Autodesk Inventor part; units mm, degrees
ref_plane "YZ Plane" through (0, 0, 0) normal (1, 0, 0) x (0, 1, 0)
ref_plane "XZ Plane" through (0, 0, 0) normal (0, 1, 0) x (-1, 0, 0)
ref_plane "XY Plane" through (0, 0, 0) normal (0, 0, 1) x (1, 0, 0)
sketch "Sketch1" plane through (0, 0, 0) normal (0, 0, 1) x (1, 0, 0)
  circle A0 centre (0, 0) radius 3.175
  circle A1 centre (0, 0) radius 1.5875
  dimension "d0" = 6.35
  dimension "d1" = 3.175
extrude "Extrusion1" add sketch "Sketch1" along normal blind 2.3813
sketch "Sketch2" plane through (0, 0, 2.3813) normal (0, 0, 1) x (1, 0, 0)
  circle A0 centre (0, 0) radius 1.905
  circle A1 centre (0, 0) radius 2.8575
  dimension "d4" = 3.81
  dimension "d5" = 5.715
extrude "Extrusion2" cut sketch "Sketch2" against normal blind 0.127
sketch "Sketch3" plane through (0, 0, 0) normal (0, 0, -1) x (-1, 0, 0)
  circle A0 centre (0, 0) radius 2.8575
  circle A1 centre (0, 0) radius 1.905
extrude "Extrusion3" cut sketch "Sketch3" against normal blind 0.127
properties part number "bearing_1_8inch" material "Stainless Steel"
Could you check a few things on this model? Use its own coordinates, in mm. A direction names the side the tool comes from. Give positions to 0.01 mm unless a question says otherwise; leave off trailing zeros. Write each loop counter-clockwise with the first axis right and the second up, starting at its lowest first coordinate (ties: lowest second). Pieces come first, ordered by that corner, then holes. Notation, with made-up numbers: (-31.5, 83.5) -> (15.5, 83.5) arc R17 ccw to (15.5, 87.5) -> close; hole circle Ø11 at (72, 55). An arc over 180 degrees is marked (long way). Answer as CSV lines item,"result". Start each with the question number.
(1) I'm going to push flat-ended pins straight in: pin 1 Ø1.7 at (x, y) = (1, -0.5) entering from -Z; pin 2 Ø1 at (y, z) = (-2, 0.5) entering from -X. Where does each tip first touch, or does it pass through?
(2) If we mould it in two halves opening along X, with no side actions, what happens to faces 1 (the face through (-0.69, 3.1, 1.17)), 2 (the face through (-1, -2, 0.127))? For each: +X half, -X half, draft (parallel to the pull), parting line (faces both ways), or undercut.
(3) Which directions (+Z, -Z, +X, -X, +Y, -Y) give clear straight access to the entire face, cutting with the end or side of a thin tool? Please do faces 3 (the face through (1, -2, 2.254)), 4 (the face through (-0.34, 1.55, 1.17)).
(4) If we section it at C-C, the plane x = 2.75: Write out the boundary of the cut face in (y, z), and give its area (3 significant figures).
(5) Please list where these lines run through material, in increasing order: line 1 (Y direction, x = 0, z = 0.05) (1 decimal); line 2 (Y direction, x = 0, z = 0.9) (1 decimal); line 3 (Z direction, x = 2.25, y = 0.75).
Answer list:
1,pin 1,"z = 0"
1,pin 2,"x = -2.8"
2,face 1,"parting line"
2,face 2,"undercut"
3,face 3,"+Z"
3,face 4,"+Z, -Z"
4,outline,"(-1.59, 0) -> (-0.78, 0) -> (-0.78, 0.13) -> (0.78, 0.13) -> (0.78, 0) -> (1.59, 0) -> (1.59, 2.38) -> (0.78, 2.38) -> (0.78, 2.25) -> (-0.78, 2.25) -> (-0.78, 2.38) -> (-1.59, 2.38) -> close"
4,area,"7.16 mm^2"
5,line 1,"-3.2 to -2.9, -1.9 to -1.6, 1.6 to 1.9, 2.9 to 3.2"
5,line 2,"-3.2 to -1.6, 1.6 to 3.2"
5,line 3,"0.13 to 2.25"
